Work out the finished part from the listing and answer in its coordinate system (mm). A direction names the side the tool comes from. Coordinates: 2 decimals unless noted, no trailing zeros. Order: outer loops, then holes, each group sorted by start corner. A loop starts at its lowest first (then second) coordinate and runs counter-clockwise, first axis right, second up. Notation, with made-up numbers: (43.25, 29.5) - (47.25, 29.5) arc R29 ccw to (47.25, 49.5) - close; hole circle Ø5 at (74, 1.5). An arc over 180 degrees is marked (long way). Answer as a JSON object with one key per item and string values. Group by question number.
1) A tool of negligible diameter and unlimited length cuts with its end or side. For faces 1 (the face through (5, 1, 9)), 2 (the face through (-2.55, 4, -9)), 3 (the face through (-0.303, 1.014, -6.133)), 4 (the face through (9, 2, 1)), from which of +Z, -Z, +X, -X, +Y, -Y can it reach the whole face along a straight path? Write none if from no direction.
2) Section A-A (z = 0) is taken. Count the separate pieces of the cut face and the enclosed holes in it, plus the area to 3 significant figures.
3) Find the intervals of material crossed by line 1 along Z through (x, y) = (0, 1.3) (3 decimals); line 2 along Z through (x, y) = (0, 0.75), in increasing order.
4) Section C-C (y = 3.5) is taken. Give the vertices of the cut face in (x, z) (3 decimals).
5) Section D-D (y = 6.5) is taken. Give the vertices of the cut face in (x, z), plus the area to 3 significant figures.
6) Each of these flat-tipped pins is pushed along its axis until it touches: P1, Ø5.5, axis at x = 1, z = -7, coming from the +Y side; P2, Ø1.8, axis at x = 8, y = 4, coming from the +Z side; P3, Ø2.5, axis at x = 9, y = 3, coming from the -Z side. Where does it stop, or does it pass through?
7) The mould has two halves that part along Z. Classify faces 5 (the face through (-2.55, 4, 9)), 6 (the face through (0, 5, 0)), 7 (the face through (0.06, 3.52, 4.95)): released by +Z, released by -Z, zero draft, split by the parting line, or undercut.
from build123d import *

# Parameters (mm, degrees)
SKETCH1_R           = 11
BOSS_EXTRUDE1_DEPTH = 1
SKETCH2_R           = 10.075
BOSS_EXTRUDE2_DEPTH = 4
CHAMFER1_SIZE       = 0.2
SKETCH3_R           = 1.4
CUT_EXTRUDE1_DEPTH  = 6
CUT_EXTRUDE2_DEPTH  = 3
SKETCH5_R           = 4.5
BOSS_EXTRUDE3_DEPTH = 2.5
SKETCH6_R           = 3
CUT_EXTRUDE3_DEPTH  = 2.5
CHAMFER2_SIZE       = 0.3


with BuildPart() as part:
    # Sketch1 → Boss-Extrude1 (new body)
    with BuildSketch(Plane(origin=(0, 0, 0), x_dir=(1, 0, 0), z_dir=(0, 1, 0))):
        Circle(SKETCH1_R)
    extrude(amount=BOSS_EXTRUDE1_DEPTH)

    # Sketch2 → Boss-Extrude2 (add)
    with BuildSketch(Plane(origin=(0, 1, 0), x_dir=(1, 0, 0), z_dir=(0, 1, 0))):
        Circle(SKETCH2_R)
    extrude(amount=BOSS_EXTRUDE2_DEPTH)

    # Chamfer1
    chamfer1_edges = [part.edges().sort_by_distance(p)[0] for p in [
        (-10.075, 5, 0),
    ]]
    chamfer(chamfer1_edges, length=CHAMFER1_SIZE)

    # Sketch3 → Cut-Extrude1 (cut, through all)
    with BuildSketch(Plane(origin=(0, 5, 0), x_dir=(1, 0, 0), z_dir=(0, 1, 0))):
        with Locations((0, 7.5)):
            Circle(SKETCH3_R)
        with Locations((7.5, 0)):
            Circle(SKETCH3_R)
        with Locations((0, -7.5)):
            Circle(SKETCH3_R)
        with Locations((-7.5, 0)):
            Circle(SKETCH3_R)
    extrude(amount=-CUT_EXTRUDE1_DEPTH, mode=Mode.SUBTRACT)

    # Sketch4 → Cut-Extrude2 (cut)
    with BuildSketch(Plane(origin=(0, 5, 0), x_dir=(1, 0, 0), z_dir=(0, 1, 0))):
        with BuildLine():
            Line((-2.55, 7.5), (-2.55, 9.746954653))
            ThreePointArc((-2.55, 9.746954653), (0, 10.075), (2.55, 9.746954653))
            Line((2.55, 9.746954653), (2.55, 7.5))
            ThreePointArc((2.55, 7.5), (0, 4.95), (-2.55, 7.5))
        make_face()
        with BuildLine():
            Line((7.5, -2.55), (9.746954653, -2.55))
            ThreePointArc((9.746954653, -2.55), (10.075, 0), (9.746954653, 2.55))
            Line((9.746954653, 2.55), (7.5, 2.55))
            ThreePointArc((7.5, 2.55), (4.95, 0), (7.5, -2.55))
        make_face()
        with BuildLine():
            Line((-2.55, -7.5), (-2.55, -9.746954653))
            ThreePointArc((-2.55, -9.746954653), (0, -10.075), (2.55, -9.746954653))
            Line((2.55, -9.746954653), (2.55, -7.5))
            ThreePointArc((2.55, -7.5), (0, -4.95), (-2.55, -7.5))
        make_face()
        with BuildLine():
            Line((-7.5, 2.55), (-9.746954653, 2.55))
            ThreePointArc((-9.746954653, 2.55), (-10.075, 0), (-9.746954653, -2.55))
            Line((-9.746954653, -2.55), (-7.5, -2.55))
            ThreePointArc((-7.5, -2.55), (-4.95, 0), (-7.5, 2.55))
        make_face()
    extrude(amount=-CUT_EXTRUDE2_DEPTH, mode=Mode.SUBTRACT)

    # Sketch5 → Boss-Extrude3 (add)
    with BuildSketch(Plane(origin=(0, 5, 0), x_dir=(1, 0, 0), z_dir=(0, 1, 0))):
        Circle(SKETCH5_R)
    extrude(amount=BOSS_EXTRUDE3_DEPTH)

    # Sketch6 → Cut-Extrude3 (cut)
    with BuildSketch(Plane(origin=(0, 7.5, 0), x_dir=(1, 0, 0), z_dir=(0, 1, 0))):
        Circle(SKETCH6_R)
    extrude(amount=-CUT_EXTRUDE3_DEPTH, mode=Mode.SUBTRACT)

    # Chamfer2
    chamfer2_edges = [part.edges().sort_by_distance(p)[0] for p in [
        (-4.5, 5, 0),
        (-4.5, 7.5, 0),
        (-3, 7.5, 0),
    ]]
    chamfer(chamfer2_edges, length=CHAMFER2_SIZE)


solid = part.part
Report:
{
 "1": {"face 1": "+Y", "face 2": "-Z, +Y", "face 3": "+Y, -Y", "face 4": "+X, +Y"},
 "2": {"separate pieces": "3", "enclosed holes": "0", "area": "68.1 mm²"},
 "3": {"line 1": "z = -10.075 to -8.9, -6.1 to 6.1, 8.9 to 10.075", "line 2": "z = -11 to -8.9, -6.1 to 6.1, 8.9 to 11"},
 "4": {"outline": "(-9.747, -2.55) arc R10.075 ccw to (-2.55, -9.747) - (-2.55, -7.5) arc R2.55 cw to (2.55, -7.5) - (2.55, -9.747) arc R10.075 ccw to (9.747, -2.55) - (7.5, -2.55) arc R2.55 cw to (7.5, 2.55) - (9.747, 2.55) arc R10.075 ccw to (2.55, 9.747) - (2.55, 7.5) arc R2.55 cw to (-2.55, 7.5) - (-2.55, 9.747) arc R10.075 ccw to (-9.747, 2.55) - (-7.5, 2.55) arc R2.55 cw to (-7.5, -2.55) - close"},
 "5": {"outline": "circle Ø9 at (0, 0); hole circle Ø6 at (0, 0)", "area": "35.3 mm²"},
 "6": {"P1": "stops at y = 7.38", "P2": "stops at z = 7.15", "P3": "stops at z = -6.44"},
 "7": {"face 5": "zero draft", "face 6": "undercut", "face 7": "released by +Z"}
}
